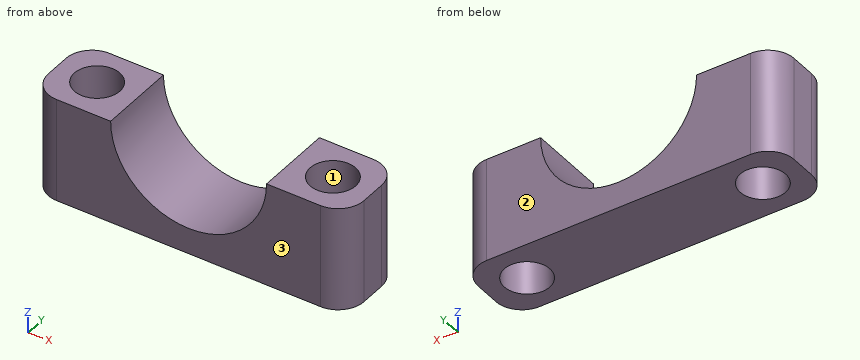
```python
from build123d import *

# Parameters (mm, degrees)
F0_W     = 24.3
F0_H     = 6
F1_DEPTH = 8
F2_R     = 6
F3_DEPTH = 6.001
F4_R     = 1.75
F5_DEPTH = 8.001
F6_R     = 2


with BuildPart() as f1:
    # F0 (on Top) → F1 (new body)
    with BuildSketch(Plane.XY):
        Rectangle(F0_W, F0_H)
    extrude(amount=F1_DEPTH)

    # F2 (on face) → F3 (cut, through all)
    with BuildSketch(Plane.XZ.offset(3)):
        with Locations((0, 8)):
            Circle(F2_R)
    extrude(amount=-F3_DEPTH, mode=Mode.SUBTRACT)

    # F4 (on face) → F5 (cut, through all)
    with BuildSketch(Plane.XY.offset(8)):
        with Locations((-9.075, 0)):
            Circle(F4_R)
        with Locations((9.075, 0)):
            Circle(F4_R)
    extrude(amount=-F5_DEPTH, mode=Mode.SUBTRACT)

    # F6
    f6_edges = [f1.edges().sort_by_distance(p)[0] for p in [
        (-12.15, -3, 4),
        (-12.15, 3, 4),
        (12.15, -3, 4),
        (12.15, 3, 4),
    ]]
    fillet(f6_edges, radius=F6_R)


solid = f1.part
```
Work out the finished part from the listing and answer in its coordinate system (mm). Face numbers are marked on the shaded views. Give positions to 0.01 mm unless a question says otherwise; leave off trailing zeros. Loops run counter-clockwise (first coordinate to the right, second up) from the corner with the lowest first, then second, coordinate; pieces in that order, holes last. Notation, with made-up numbers: M 44,21 L 79,21 A35 ccw 79,57 Z; hole C -31.75,11 d5. An arc over 180 degrees is marked long. One line per item, written item: value. Start each with the question number.
1. Find section B-B (z = 5.5). Give the vertices of the cut face in (x, y) (3 decimals).
2. Each of these flat-tipped pins is pushed along its axis until it touches: P1, Ø3, axis at x = 9.075, y = 0, coming from the +Z side; P2, Ø2, axis at x = 0.5, y = 2, coming from the +Z side. Where does it stop, or does it pass through?
3. Find section D-D (x = 0). Give the vertices of the cut face in (y, z), and give its area (3 significant figures).
4. Find section C-C (z = 1). Give the vertices of the cut face in (x, y) (3 decimals), and give its area (3 significant figures).
5. Determine the mould class of the marked faces 1, 2 and 3 for opening direction Y: released by +Y, released by -Y, zero draft, split by the parting line, or undercut.
6. Find the intervals of material crossed by probe 1 along Y at (x, z) = (-9, 5.5); probe 2 along Y at (x, z) = (-10.5, 6.75); probe 3 along X at (y, z) = (2.25, 3.25), in increasing order.
7. Find section A-A (y = 0). Give the vertices of the cut face in (x, z) (3 decimals), and give its area (3 significant figures).
Reported:
1. outline: M -12.15,-1 A2 ccw -10.15,-3 L -5.454,-3 L -5.454,3 L -10.15,3 A2 ccw -12.15,1 Z; M 5.454,-3 L 10.15,-3 A2 ccw 12.15,-1 L 12.15,1 A2 ccw 10.15,3 L 5.454,3 Z; hole C -9.075,0 d3.5; hole C 9.075,0 d3.5
2. P1: passes through
2. P2: stops at z = 2.19
3. outline: M -3,0 L 3,0 L 3,2 L -3,2 Z
3. area: 12.0 mm²
4. outline: M -12.15,-1 A2 ccw -10.15,-3 L 10.15,-3 A2 ccw 12.15,-1 L 12.15,1 A2 ccw 10.15,3 L -10.15,3 A2 ccw -12.15,1 Z; hole C -9.075,0 d3.5; hole C 9.075,0 d3.5
4. area: 123 mm²
5. face 1: undercut
5. face 2: released by +Y
5. face 3: released by -Y
6. probe 1: y = -3 to -1.75, 1.75 to 3
6. probe 2: y = -2.97 to -1.02, 1.02 to 2.97
6. probe 3: x = -11.71 to -3.67, 3.67 to 11.71
7. outline: M -12.15,0 L -10.825,0 L -10.825,8 L -12.15,8 Z; M -7.325,0 L 7.325,0 L 7.325,8 L 6,8 A6 cw -6,8 L -7.325,8 Z; M 10.825,0 L 12.15,0 L 12.15,8 L 10.825,8 Z
7. area: 81.9 mm²
